```python
from build123d import *

# Parameters (mm, degrees)
F0_W     = 7.5
F0_H     = 7.5
F0_W_2   = 0.1
F0_H_2   = 0.1
F0_H_3   = 2.9
F0_W_3   = 0.3
F0_W_4   = 2.9
F1_DEPTH = 1.8
F2_W     = 0.6
F2_H     = 7.5
F3_DEPTH = 1.2
F4_W     = 0.6
F4_H     = 7.5
F5_DEPTH = 1.2
F7_DEPTH = 1.2
F9_DEPTH = 1.2
F10_R    = 1
F11_R    = 0.59999


# Not quite as in the source:
# - a fillet or chamfer is up to 0.001 mm smaller than in the source, because OpenCascade refuses the exact size


with BuildPart() as f1:
    # F0 (on Front) → F1 (new body)
    with BuildSketch(Plane.XZ):
        with Locations((-0.15, 3.15)):
            Rectangle(F0_W, F0_H)
        Polygon((-0.3, 3), (-0.3, 2.9), (-0.3, 0), (-0.4, 0), (-3.3, 0), (-3.3, 2.9), (-3.3, 3), (-0.4, 3), align=None, mode=Mode.SUBTRACT)
        Polygon((0.1, 0), (0, 0), (0, 2.9), (0, 3), (0.1, 3), (3, 3), (3, 2.9), (3, 0), align=None, mode=Mode.SUBTRACT)
        Polygon((0.1, 3.3), (0, 3.3), (-0.3, 3.3), (-0.4, 3.3), (-3.3, 3.3), (-3.3, 3.4), (-3.3, 6.3), (-0.4, 6.3), (-0.3, 6.3), (-0.3, 3.4), (0, 3.4), (0, 6.3), (0.1, 6.3), (3, 6.3), (3, 3.4), (3, 3.3), align=None, mode=Mode.SUBTRACT)
        with Locations((-0.35, 3.35)):
            Rectangle(F0_W_2, F0_H_2)
        with Locations((-0.35, 4.85)):
            Rectangle(F0_W_2, F0_H_3)
        with Locations((0.05, 3.35)):
            Rectangle(F0_W_2, F0_H_2)
        with Locations((0.05, 4.85)):
            Rectangle(F0_W_2, F0_H_3)
        with Locations((-0.15, 3.35)):
            Rectangle(F0_W_3, F0_H_2)
        with Locations((-1.85, 3.35)):
            Rectangle(F0_W_4, F0_H_2)
        with Locations((1.55, 3.35)):
            Rectangle(F0_W_4, F0_H_2)
        with Locations((1.55, 2.95)):
            Rectangle(F0_W_4, F0_H_2)
        with Locations((-1.85, 2.95)):
            Rectangle(F0_W_4, F0_H_2)
        with Locations((-0.35, 1.45)):
            Rectangle(F0_W_2, F0_H_3)
        with Locations((0.05, 1.45)):
            Rectangle(F0_W_2, F0_H_3)
        with Locations((0.05, 2.95)):
            Rectangle(F0_W_2, F0_H_2)
        with Locations((-0.35, 2.95)):
            Rectangle(F0_W_2, F0_H_2)
    extrude(amount=F1_DEPTH)

    # F2 (on face) → F3 (join)
    with BuildSketch(Plane(origin=(-3.9, 0, 0), x_dir=(0, -1, 0), z_dir=(-1, 0, 0))):
        with Locations((1.5, 3.15)):
            Rectangle(F2_W, F2_H)
    extrude(amount=F3_DEPTH)

    # F4 (on face) → F5 (join)
    with BuildSketch(Plane.YZ.offset(3.6)):
        with Locations((-1.5, 3.15)):
            Rectangle(F4_W, F4_H)
    extrude(amount=F5_DEPTH)

    # F6 (on face) → F7 (join)
    with BuildSketch(Plane.XY.offset(6.9)):
        Polygon((-5.1, -1.2), (-5.1, -1.2278293749), (-5.1, -1.8), (4.8, -1.8), (4.8, -1.2), (3.6, -1.2), (-3.9, -1.2), align=None)
    extrude(amount=F7_DEPTH)

    # F8 (on face) → F9 (join)
    with BuildSketch(Plane(origin=(0, 0, -0.6), x_dir=(1, 0, 0), z_dir=(0, 0, -1))):
        Polygon((3.6, 1.2), (4.8, 1.2), (4.8, 1.8), (-5.1, 1.8), (-5.1, 1.2), (-3.9, 1.2), align=None)
    extrude(amount=F9_DEPTH)

    # F10
    f10_edges = [f1.edges().sort_by_distance(p)[0] for p in [
        (-5.1, -1.5, -1.8),
        (4.8, -1.5, -1.8),
        (4.8, -1.5, 8.1),
        (-5.1, -1.5, 8.1),
    ]]
    fillet(f10_edges, radius=F10_R)

    # F11 (radius 0.6 in the source; OpenCascade refuses exactly that, so slightly less here)
    f11_edges = [f1.edges().sort_by_distance(p)[0] for p in [
        (-5.1, -1.8, 3.15),
    ]]
    fillet(f11_edges, radius=F11_R)


solid = f1.part
```
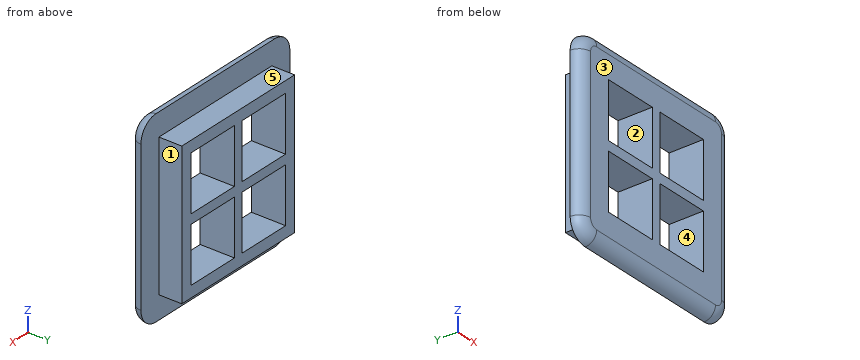
Part model, mm, in its own coordinate system. Face numbers are marked on the shaded views. A direction names the side the tool comes from. Coordinates: 2 decimals unless noted, no trailing zeros. Order: outer loops, then holes, each group sorted by start corner. A loop starts at its lowest first (then second) coordinate and runs counter-clockwise, first axis right, second up. Notation, with made-up numbers: (-7, 23) -> (33, 23) arc R30 cw to (33, 58) -> close; hole circle Ø9 at (76, -23). An arc over 180 degrees is marked (long way). Put each result on its own line as item: value. Start each with the question number.
(1) Which spindle directions (+Z, -Z, +X, -X, +Y, -Y) get a long thin tool onto all of the face, cutting with end or side? Do the marked faces 1 and 2. Say none if no direction does.
(2) Pin check, flat tips, straight feed: pin 1 Ø0.9 at (x, y) = (-2, -1) entering from +Z; pin 2 Ø0.9 at (x, y) = (1.5, -0.5) entering from -Z. Stop position of each tip, or through.
(3) Band-saw the part on A-A (x = 2). Count the separate pieces of the cut face and the enclosed holes in it, then the cut area to 3 significant figures.
(4) Band-saw the part on B-B (y = -0.2). Give the cut face in (x, z).
(5) Probe line 1 along Z through (x, y) = (-2.75, -0.1); line 2 along Z through (x, y) = (1.5, -1.25); line 3 along X through (y, z) = (-0.2, 6.25). List the from-to ranges inside material, lowest first. Write a range as [from, to].
(6) Mould opens along Z. For the marked faces 3, 4 and 5 say: pulls with the +Z half, pulls with the -Z half, needs draft (parallel to the pull), parting line crosses it, or undercut.
Determined:
1. face 1: +Z, -Z, +X, +Y
1. face 2: +Y, -Y
2. pin 1: stops at z = 8.1
2. pin 2: stops at z = -0.6
3. separate pieces: 3
3. enclosed holes: 0
3. area: 4.35 mm²
4. outline: (-3.9, -0.6) -> (3.6, -0.6) -> (3.6, 6.9) -> (-3.9, 6.9) -> close; hole (-3.3, 0) -> (-0.4, 0) -> (-0.4, 2.9) -> (-3.3, 2.9) -> close; hole (-3.3, 3.4) -> (-0.4, 3.4) -> (-0.4, 6.3) -> (-3.3, 6.3) -> close; hole (0.1, 0) -> (3, 0) -> (3, 2.9) -> (0.1, 2.9) -> close; hole (0.1, 3.4) -> (3, 3.4) -> (3, 6.3) -> (0.1, 6.3) -> close
5. line 1: z = [-0.6, 0], [2.9, 3.4], [6.3, 6.9]
5. line 2: z = [-1.8, 0], [2.9, 3.4], [6.3, 8.1]
5. line 3: x = [-3.9, -3.3], [-0.4, 0.1], [3, 3.6]
6. face 3: needs draft
6. face 4: undercut
6. face 5: pulls with the +Z half
